Part model, mm, in its own coordinate system. Face numbers are marked on the shaded views. A direction names the side the tool comes from. Coordinates: 2 decimals unless noted, no trailing zeros. Loops run counter-clockwise (first coordinate to the right, second up) from the corner with the lowest first, then second, coordinate; pieces in that order, holes last. Notation, with made-up numbers: (0.5, -30) -> (10.5, -30) arc R21 cw to (10.5, -15) -> close; hole circle Ø3 at (46.5, -5.5). An arc over 180 degrees is marked (long way). One line per question, with ' | ' between items. Start each with the question number.
1) 3-axis set-ups, long thin cutter, end or side, ignore diameter. For the marked faces 1 and 2: which of +Z, -Z, +X, -X, +Y, -Y reach the whole face in a straight line?
2) Cut at A-A (z = -11). List the corners of the cut face in (x, y).
3) Probe L1, parallel to X at y = -18.75, z = -7.5; L2, parallel to X at y = -2, z = 4; L3, parallel to Z at x = 24.5, y = -9. List the from-to ranges inside material, lowest first. Write a range as from..to.
4) Cut at D-D (x = 52). List the corners of the cut face in (y, z), plus the area to 3 significant figures.
5) Drop flat-ended pins along their axis: pin 1 (12 mm diameter, centred on y = -4.5, z = -29.5, fed in from -X); pin 2 (1.8 mm diameter, centred on x = 1.12, z = -23.86, fed in from -Y) (1 decimal); pin 3 (7.5 mm diameter, centred on x = -19, y = -15, fed in from +Z); pin 4 (8 mm diameter, centred on y = -15, z = -18, fed in from +X). Give the stop position or say it passes through.
6) Two-plate mould, pull along Z, no slides. Class the marked faces 3, 4 and 5: released by +Z, released by -Z, zero draft, split by the parting line, or undercut.
7) Cut at C-C (y = -5.25). List the corners of the cut face in (x, z) (3 decimals).
8) Cut at B-B (x = -12). List the corners of the cut face in (y, z), plus the area to 3 significant figures.
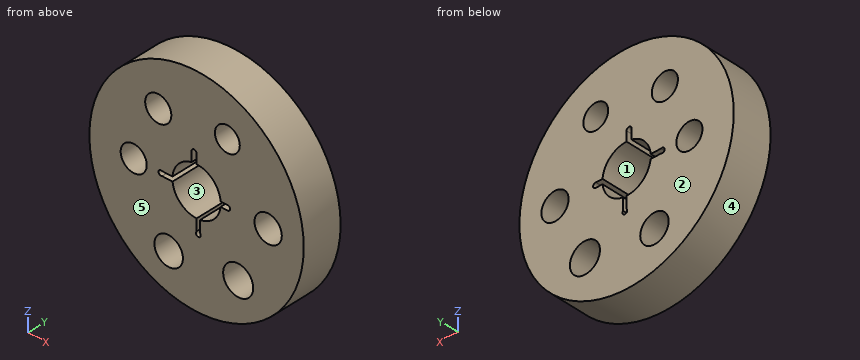
from build123d import *

# Parameters (mm, degrees)
F0_R     = 68.2142
F0_R_2   = 9.06213
F0_R_3   = 9.570677
F0_R_4   = 8.295327
F0_R_5   = 8.314873
F0_R_6   = 15.377147
F0_R_7   = 8.676921
F0_R_8   = 7.903736
F1_DEPTH = 25.4
F3_DEPTH = 25.401
F4_W     = 2.246405
F4_H     = 9.179381
F5_DEPTH = 25.401


with BuildPart() as f1:
    # F0 (on Front) → F1 (new body)
    with BuildSketch(Plane.XZ):
        Circle(F0_R)
        with Locations((-17.750563, -42.127229)):
            Circle(F0_R_2, mode=Mode.SUBTRACT)
        with Locations((26.49338, -38.153224)):
            Circle(F0_R_3, mode=Mode.SUBTRACT)
        with Locations((-40.004998, 0)):
            Circle(F0_R_4, mode=Mode.SUBTRACT)
        with Locations((-24.373908, 35.498366)):
            Circle(F0_R_5, mode=Mode.SUBTRACT)
        Circle(F0_R_6, mode=Mode.SUBTRACT)
        with Locations((45.568611, 0)):
            Circle(F0_R_7, mode=Mode.SUBTRACT)
        with Locations((19.605096, 38.677573)):
            Circle(F0_R_8, mode=Mode.SUBTRACT)
    extrude(amount=F1_DEPTH)

    # F2 (on face) → F3 (cut, through all)
    with BuildSketch(Plane.XZ.offset(25.4)):
        Polygon((-3.167718, 21.456879), (-3.167718, 15.047332), (0, 15.377147), (0, 21.456879), align=None)
        with BuildLine():
            ThreePointArc((0, 21.456879), (-1.583859, 23.040738), (-3.167718, 21.456879))
            Line((-3.167718, 21.456879), (0, 21.456879))
        make_face()
    extrude(amount=-F3_DEPTH, mode=Mode.SUBTRACT)

    # F4 (on face) → F5 (cut, through all)
    with BuildSketch(Plane.XZ.offset(25.4)):
        with BuildLine():
            Line((19.603778, 1.377483), (15.315325, 1.377483))
            Line((15.315325, 1.377483), (13.762355, 0))
            Line((13.762355, 0), (15.281475, -1.712651))
            Line((15.281475, -1.712651), (19.770676, -1.712651))
            ThreePointArc((19.770676, -1.712651), (21.317995, -0.079506), (19.603778, 1.377483))
        make_face()
        Polygon((-13.441991, 1.215727), (-13.775786, 1.215727), (-13.775786, 0), (-13.775786, -1.621536), align=None)
        Polygon((-13.775786, 0), (-13.775786, 1.215727), (-21.95378, 1.215727), (-21.95378, -1.621536), (-13.775786, -1.621536), align=None)
        with BuildLine():
            Line((-21.95378, -1.621536), (-21.95378, 1.215727))
            ThreePointArc((-21.95378, 1.215727), (-24.235262, -0.202904), (-21.95378, -1.621536))
        make_face()
        with Locations((1.123202, -18.22787)):
            Rectangle(F4_W, F4_H)
        with BuildLine():
            Line((2.246405, -22.81756), (0, -22.81756))
            ThreePointArc((0, -22.81756), (1.123202, -25.390364), (2.246405, -22.81756))
        make_face()
    extrude(amount=-F5_DEPTH, mode=Mode.SUBTRACT)


solid = f1.part
Reported:
1) face 1: +Y, -Y | face 2: +Z, -Z, +X, -X, +Y
2) outline: (-67.32, -25.4) -> (-10.75, -25.4) -> (-10.75, 0) -> (-67.32, 0) -> close; (10.75, -25.4) -> (67.32, -25.4) -> (67.32, 0) -> (10.75, 0) -> close
3) L1: x = -67.8..-43.55, -36.46..-13.42, 13.42..41.21, 49.93..67.8 | L2: x = -68.1..-47.27, -32.74..-14.85, 14.85..37.87, 53.27..68.1 | L3: z = -63.66..-47.51, -28.79..32.47, 44.88..63.66
4) outline: (-25.4, -44.15) -> (0, -44.15) -> (0, -5.82) -> (-25.4, -5.82) -> close; (-25.4, 5.82) -> (0, 5.82) -> (0, 44.15) -> (-25.4, 44.15) -> close | area: 1,950 mm²
5) pin 1: stops at x = -64.04 | pin 2: passes through | pin 3: stops at z = 66.49 | pin 4: stops at x = 66.76
6) face 3: undercut | face 4: split by the parting line | face 5: zero draft
7) outline: circle Ø136.428 at (0, 0); hole circle Ø16.591 at (-40.005, 0); hole circle Ø16.63 at (-24.374, 35.498); hole circle Ø18.124 at (-17.751, -42.127); hole (-21.954, -1.622) -> (-15.291, -1.622) arc R15.377 ccw to (0, -15.377) -> (0, -22.818) arc R1.532 ccw (long way) to (2.246, -22.818) -> (2.246, -15.212) arc R15.377 ccw to (15.281, -1.713) -> (19.771, -1.713) arc R1.55 ccw (long way) to (19.604, 1.377) -> (15.315, 1.377) arc R15.377 ccw to (0, 15.377) -> (0, 21.457) arc R1.584 ccw to (-3.168, 21.457) -> (-3.168, 15.047) arc R15.377 ccw to (-15.329, 1.216) -> (-21.954, 1.216) arc R1.582 ccw (long way) to start; hole circle Ø15.807 at (19.605, 38.678); hole circle Ø19.141 at (26.493, -38.153); hole circle Ø17.354 at (45.569, 0)
8) outline: (-25.4, -67.15) -> (0, -67.15) -> (0, -49.13) -> (-25.4, -49.13) -> close; (-25.4, -35.12) -> (0, -35.12) -> (0, -9.62) -> (-25.4, -9.62) -> close; (-25.4, 9.62) -> (0, 9.62) -> (0, 67.15) -> (-25.4, 67.15) -> close | area: 2,570 mm²
